Work out the finished part from the listing and answer in its coordinate system (mm). Give positions to 0.01 mm unless a question says otherwise; leave off trailing zeros. Loops run counter-clockwise (first coordinate to the right, second up) from the corner with the lowest first, then second, coordinate; pieces in that order, holes last. Notation, with made-up numbers: (22, 88.25) - (61, 88.25) arc R25 ccw to (61, 119.25) - close; hole circle Ø8 at (31.5, 18). An arc over 180 degrees is marked (long way). One line per item, written item: value.
from build123d import *

# Parameters (mm, degrees)
SKETCH1_W           = 65.5
SKETCH1_H           = 65.5
SKETCH1_R           = 3.5
SKETCH1_R_2         = 2.5
BOSS_EXTRUDE1_DEPTH = 3


with BuildPart() as part:
    # Sketch1 → Boss-Extrude1 (new body)
    with BuildSketch(Plane.XY):
        Rectangle(SKETCH1_W, SKETCH1_H)
        with Locations((-19.85, 20)):
            Circle(SKETCH1_R, mode=Mode.SUBTRACT)
        with Locations((-19.85, 10)):
            Circle(SKETCH1_R_2, mode=Mode.SUBTRACT)
        with Locations((-19.85, 0)):
            Circle(SKETCH1_R_2, mode=Mode.SUBTRACT)
        with Locations((-19.85, -10)):
            Circle(SKETCH1_R_2, mode=Mode.SUBTRACT)
        with Locations((-19.85, -20)):
            Circle(SKETCH1_R, mode=Mode.SUBTRACT)
        with Locations(Location((19.85, -20, 0), (0, 0, 180))):
            Circle(SKETCH1_R, mode=Mode.SUBTRACT)
        with Locations(Location((19.85, -10, 0), (0, 0, 180))):
            Circle(SKETCH1_R_2, mode=Mode.SUBTRACT)
        with Locations(Location((19.85, 0, 0), (0, 0, 180))):
            Circle(SKETCH1_R_2, mode=Mode.SUBTRACT)
        with Locations(Location((19.85, 10, 0), (0, 0, 180))):
            Circle(SKETCH1_R_2, mode=Mode.SUBTRACT)
        with Locations(Location((19.85, 20, 0), (0, 0, 180))):
            Circle(SKETCH1_R, mode=Mode.SUBTRACT)
        Circle(SKETCH1_R_2, mode=Mode.SUBTRACT)
        with Locations((10, 0)):
            Circle(SKETCH1_R_2, mode=Mode.SUBTRACT)
        with Locations((-10, 0)):
            Circle(SKETCH1_R_2, mode=Mode.SUBTRACT)
        with Locations((0, 10)):
            Circle(SKETCH1_R_2, mode=Mode.SUBTRACT)
        with Locations((0, -10)):
            Circle(SKETCH1_R_2, mode=Mode.SUBTRACT)
        with BuildLine():
            Line((-23.1, 29.2), (-16.6, 29.2))
            ThreePointArc((-16.6, 29.2), (-15.1, 27.7), (-16.6, 26.2))
            Line((-16.6, 26.2), (-23.1, 26.2))
            ThreePointArc((-23.1, 26.2), (-24.6, 27.7), (-23.1, 29.2))
        make_face(mode=Mode.SUBTRACT)
        with BuildLine():
            Line((-23.1, -26.2), (-16.6, -26.2))
            ThreePointArc((-16.6, -26.2), (-15.1, -27.7), (-16.6, -29.2))
            Line((-16.6, -29.2), (-23.1, -29.2))
            ThreePointArc((-23.1, -29.2), (-24.6, -27.7), (-23.1, -26.2))
        make_face(mode=Mode.SUBTRACT)
        with BuildLine():
            Line((-3.25, 29.2), (3.25, 29.2))
            ThreePointArc((3.25, 29.2), (4.75, 27.7), (3.25, 26.2))
            Line((3.25, 26.2), (-3.25, 26.2))
            ThreePointArc((-3.25, 26.2), (-4.75, 27.7), (-3.25, 29.2))
        make_face(mode=Mode.SUBTRACT)
        with BuildLine():
            Line((-3.25, -29.2), (3.25, -29.2))
            ThreePointArc((3.25, -29.2), (4.75, -27.7), (3.25, -26.2))
            Line((3.25, -26.2), (-3.25, -26.2))
            ThreePointArc((-3.25, -26.2), (-4.75, -27.7), (-3.25, -29.2))
        make_face(mode=Mode.SUBTRACT)
        with BuildLine():
            Line((23.1, -26.2), (16.6, -26.2))
            ThreePointArc((16.6, -26.2), (15.1, -27.7), (16.6, -29.2))
            Line((16.6, -29.2), (23.1, -29.2))
            ThreePointArc((23.1, -29.2), (24.6, -27.7), (23.1, -26.2))
        make_face(mode=Mode.SUBTRACT)
        with BuildLine():
            Line((23.1, 29.2), (16.6, 29.2))
            ThreePointArc((16.6, 29.2), (15.1, 27.7), (16.6, 26.2))
            Line((16.6, 26.2), (23.1, 26.2))
            ThreePointArc((23.1, 26.2), (24.6, 27.7), (23.1, 29.2))
        make_face(mode=Mode.SUBTRACT)
    extrude(amount=BOSS_EXTRUDE1_DEPTH)


solid = part.part
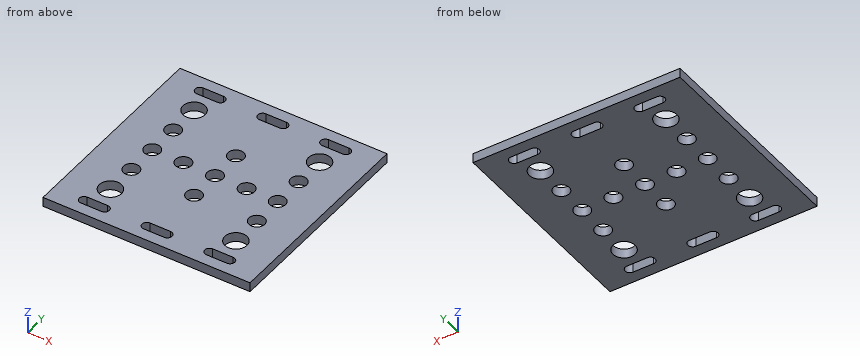
1. Section A-A (y = 27.7) is taken. Write down the section's boundary in (x, z).
Output:
outline: (-32.75, 0) - (-24.6, 0) - (-24.6, 3) - (-32.75, 3) - close; (-15.1, 0) - (-4.75, 0) - (-4.75, 3) - (-15.1, 3) - close; (4.75, 0) - (15.1, 0) - (15.1, 3) - (4.75, 3) - close; (24.6, 0) - (32.75, 0) - (32.75, 3) - (24.6, 3) - close
2. Section B-B (x = 0) is taken. Write down the section's boundary in (y, z), and give its area (4 significant figures).
Output:
outline: (-32.75, 0) - (-29.2, 0) - (-29.2, 3) - (-32.75, 3) - close; (-26.2, 0) - (-12.5, 0) - (-12.5, 3) - (-26.2, 3) - close; (-7.5, 0) - (-2.5, 0) - (-2.5, 3) - (-7.5, 3) - close; (2.5, 0) - (7.5, 0) - (7.5, 3) - (2.5, 3) - close; (12.5, 0) - (26.2, 0) - (26.2, 3) - (12.5, 3) - close; (29.2, 0) - (32.75, 0) - (32.75, 3) - (29.2, 3) - close
area: 133.5 mm²
3. A flat-ended cylindrical pin translates along its axis: pin 1 Ø8 at (x, y) = (0, 0) entering from -Z. Find the tip coordinate at first contact, or state that the pin passes through.
Output:
pin 1: stops at z = 0
4. Section D-D (y = 10) is taken. Write down the section's boundary in (x, z).
Output:
outline: (-32.75, 0) - (-22.35, 0) - (-22.35, 3) - (-32.75, 3) - close; (-17.35, 0) - (-2.5, 0) - (-2.5, 3) - (-17.35, 3) - close; (2.5, 0) - (17.35, 0) - (17.35, 3) - (2.5, 3) - close; (22.35, 0) - (32.75, 0) - (32.75, 3) - (22.35, 3) - close
5. Section C-C (x = 21) is taken. Count the separate pieces of the cut face and the enclosed holes in it, and give its area (3 significant figures).
Output:
separate pieces: 8
enclosed holes: 0
area: 98.9 mm²
6. Find the intervals of material crossed by line 1 along Y through (x, z) = (0, 1.95); line 2 along Y through (x, z) = (-17, 0.45); line 3 along Y through (x, z) = (-2, 1.55), in increasing order.
Output:
line 1: y = -32.75 to -29.2, -26.2 to -12.5, -7.5 to -2.5, 2.5 to 7.5, 12.5 to 26.2, 29.2 to 32.75
line 2: y = -32.75 to -29.2, -26.2 to -22.03, -17.97 to 17.97, 22.03 to 26.2, 29.2 to 32.75
line 3: y = -32.75 to -29.2, -26.2 to -11.5, -8.5 to -1.5, 1.5 to 8.5, 11.5 to 26.2, 29.2 to 32.75
